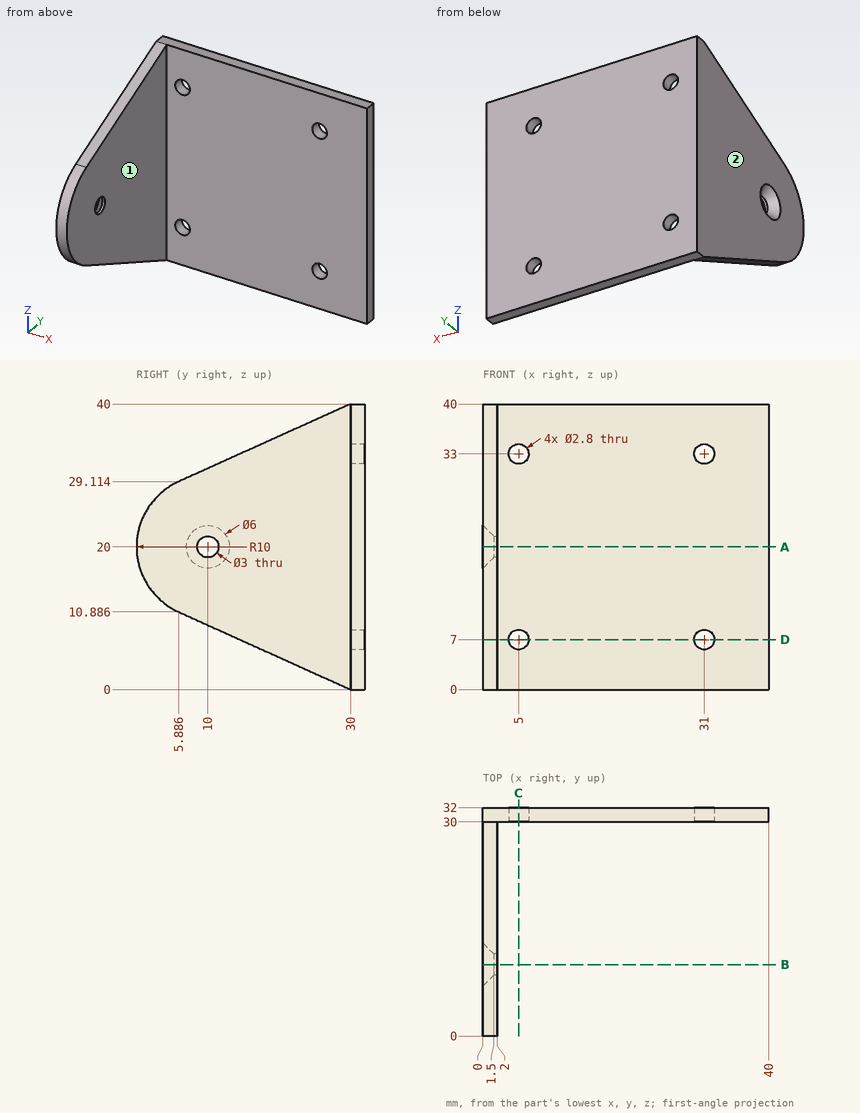
Could you check a few things on this drawing? It's one solid part, dimensions in mm from its lowest x, y, z. A direction names the side the tool comes from. Round coordinates to 2 decimals unless told otherwise and drop trailing zeros. Loops run counter-clockwise (first coordinate to the right, second up) from the corner with the lowest first, then second, coordinate; pieces in that order, holes last.
Q1. Please list where these lines run through material, in increasing order: L1, parallel to X at y = 31, z = 7; L2, parallel to X at y = 7.5, z = 22; L3, parallel to Y at x = 10.5, z = 7.5.
Q2. I want a section at C-C (x = 5). Write out the boundary of the cut face in (y, z).
Q3. For P1, Ø12, axis at x = 13.5, y = 6, coming from the -Z side; P2, Ø15, axis at y = 9.5, z = 21, coming from the +X side; P3, Ø4.5, axis at x = 31, z = 7, coming from the -Y side; P4, Ø4, axis at y = 10, z = 20, coming from the -X side, each with a flat end and sliding along its axis, tell me the tip position at first contact or that it passes through.
Q4. On a 3-axis mill with a long thin cutter (end or side, diameter ignored), from which of +Z, -Z, +X, -X, +Y, -Y can I reach the whole of each face in a straight line? I mean the marked faces 1 and 2. Say none if no direction works.
Q5. I want a section at D-D (z = 7). Write out the boundary of the cut face in (x, y).
Q6. I want a section at A-A (z = 20). Write out the boundary of the cut face in (x, y), and give its area (3 significant figures).
Q7. I want a section at B-B (y = 10). Write out the boundary of the cut face in (x, z).
Answer below:
1. L1: x = 0 to 3.6, 6.4 to 29.6, 32.4 to 40
1. L2: x = 0 to 2
1. L3: y = 30 to 32
2. outline: (30, 0) - (32, 0) - (32, 5.6) - (30, 5.6) - close; (30, 8.4) - (32, 8.4) - (32, 31.6) - (30, 31.6) - close; (30, 34.4) - (32, 34.4) - (32, 40) - (30, 40) - close
3. P1: passes through
3. P2: stops at x = 2
3. P3: stops at y = 30
3. P4: stops at x = 1
4. face 1: +Z, -Z, +X, -Y
4. face 2: +Z, -Z, -X, +Y, -Y
5. outline: (0, 14.49) - (2, 14.49) - (2, 30) - (3.6, 30) - (3.6, 32) - (0, 32) - close; (6.4, 30) - (29.6, 30) - (29.6, 32) - (6.4, 32) - close; (32.4, 30) - (40, 30) - (40, 32) - (32.4, 32) - close
6. outline: (0, 0) - (2, 0) - (2, 8.5) - (1.5, 8.5) - (0, 7) - close; (0, 13) - (1.5, 11.5) - (2, 11.5) - (2, 30) - (40, 30) - (40, 32) - (0, 32) - close
6. area: 132 mm2
7. outline: (0, 9.03) - (2, 9.03) - (2, 18.5) - (1.5, 18.5) - (0, 17) - close; (0, 23) - (1.5, 21.5) - (2, 21.5) - (2, 30.97) - (0, 30.97) - close
